Can you work these out from the model? Positions are in its coordinate system, mm. A direction names the side the tool comes from. Give positions to 0.01 mm unless a question says otherwise; leave off trailing zeros. Write each loop counter-clockwise with the first axis right and the second up, starting at its lowest first coordinate (ties: lowest second). Pieces come first, ordered by that corner, then holes. Notation, with made-up numbers: (5, -28) -> (48, -28) arc R15 ccw to (48, -20) -> close; hole circle Ø10 at (45.5, 88). An arc over 180 degrees is marked (long way). One line per item, written item: value.
from build123d import *

# Parameters (mm, degrees)
BOSS_EXTRUDE1_DEPTH     = 2.54
CUT_EXTRUDE1_DEPTH      = 60.34583774
CUT_EXTRUDE1_DEPTH_BACK = 60.34583774
SKETCH3_R               = 1.0922
SKETCH3_R_2             = 1.27
SKETCH3_R_3             = 1.016
SKETCH3_W               = 7.493
SKETCH3_H               = 35.56
SKETCH3_W_2             = 21.082
SKETCH3_H_2             = 21.59


with BuildPart() as part:
    # Sketch2 → Boss-Extrude1 (new body)
    with BuildSketch(Plane(origin=(0, 0, 0), x_dir=(1, 0, 0), z_dir=(0, 1, 0))):
        with BuildLine():
            Line((48.006, 34.798), (-48.006, 34.798))
            Line((-48.006, 34.798), (-48.006, -3.048))
            add(Edge.make_bspline(
                [(-48.006, -3.048), (-48.006, -45.381333333), (48.006, -45.381333333), (48.006, -3.048)],
                knots=[0, 0, 0, 0, 1, 1, 1, 1], degree=3))
            Line((48.006, -3.048), (48.006, 34.798))
        make_face()
    extrude(amount=BOSS_EXTRUDE1_DEPTH)

    # Sketch3 → Cut-Extrude1 (cut, two sides: drawn at the far end of the back side and taken through both)
    with BuildSketch(Plane(origin=(0, 2.54, 0), x_dir=(1, 0, 0), z_dir=(0, 1, 0)).offset(-CUT_EXTRUDE1_DEPTH_BACK)):
        with Locations(Location((-30.861, 23.4696, 0), (0, 0, 270))):
            Circle(SKETCH3_R)
        with Locations(Location((-30.861, 5.4864, 0), (0, 0, 270))):
            Circle(SKETCH3_R)
        with Locations(Location((-30.226, 30.988, 0), (0, 0, 270))):
            Circle(SKETCH3_R_2)
        with Locations(Location((30.861, 5.4864, 0), (0, 0, 90))):
            Circle(SKETCH3_R)
        with Locations(Location((30.861, 23.4696, 0), (0, 0, 90))):
            Circle(SKETCH3_R)
        with Locations(Location((-30.226, -22.352, 0), (0, 0, 270))):
            Circle(SKETCH3_R_2)
        with Locations(Location((30.226, -22.352, 0), (0, 0, 90))):
            Circle(SKETCH3_R_2)
        with Locations(Location((30.226, 30.988, 0), (0, 0, 90))):
            Circle(SKETCH3_R_2)
        with Locations(Location((-7.747, -22.606, 0), (0, 0, 270))):
            Circle(SKETCH3_R_3)
        with Locations(Location((7.747, -22.606, 0), (0, 0, 90))):
            Circle(SKETCH3_R_3)
        with Locations(Location((-20.828, 30.226, 0), (0, 0, 270))):
            Circle(SKETCH3_R_2)
        with Locations(Location((-20.828, -28.194, 0), (0, 0, 270))):
            Circle(SKETCH3_R_2)
        with Locations(Location((20.828, -28.194, 0), (0, 0, 90))):
            Circle(SKETCH3_R_2)
        with Locations(Location((20.828, 30.226, 0), (0, 0, 90))):
            Circle(SKETCH3_R_2)
        with Locations((-41.7195, 14.478)):
            Rectangle(SKETCH3_W, SKETCH3_H)
        with Locations((41.7195, 14.478)):
            Rectangle(SKETCH3_W, SKETCH3_H)
        with Locations((0, 14.859)):
            Rectangle(SKETCH3_W_2, SKETCH3_H_2)
    extrude(amount=CUT_EXTRUDE1_DEPTH + CUT_EXTRUDE1_DEPTH_BACK, mode=Mode.SUBTRACT)


solid = part.part
1) We'd pull the mould along Z, two halves only. Please class faces 3 (the face through (-6.74, 1.25, 22.47)), 4 (the face through (-31.927, 1.252, -5.723)), 5 (the face through (-1, 0, 5)): released by +Z, released by -Z, zero draft, split by the parting line, or undercut.
Answer list:
face 3: undercut
face 4: undercut
face 5: zero draft
2) If we section it at B-B (z = -16): Write out the boundary of the cut face in (x, y), and give its area (3 significant figures).
Answer list:
outline: (-48.01, 0) -> (-45.47, 0) -> (-45.47, 2.54) -> (-48.01, 2.54) -> close; (-37.97, 0) -> (-10.54, 0) -> (-10.54, 2.54) -> (-37.97, 2.54) -> close; (10.54, 0) -> (37.97, 0) -> (37.97, 2.54) -> (10.54, 2.54) -> close; (45.47, 0) -> (48.01, 0) -> (48.01, 2.54) -> (45.47, 2.54) -> close
area: 152 mm^2
3) If we section it at C-C (y = 0.9): State how many separate pieces and enclosed holes the cut face has, and give its area (3 significant figures).
Answer list:
separate pieces: 1
enclosed holes: 17
area: 5,020 mm^2
4) I need wall thicknesses on L1, parallel to X at y = 1.85, z = -22; L2, parallel to X at y = 2.1, z = -23.5; L3, parallel to X at y = 1, z = -28. Which ranges of each line are inside material? Lowest first, please.
Answer list:
L1: x = -48.01 to -45.47, -37.97 to -10.54, 10.54 to 37.97, 45.47 to 48.01
L2: x = -48.01 to -45.47, -37.97 to -31.95, -29.77 to -10.54, 10.54 to 29.77, 31.95 to 37.97, 45.47 to 48.01
L3: x = -48.01 to -45.47, -37.97 to 37.97, 45.47 to 48.01
5) If we section it at A-A (z = -3): Write out the boundary of the cut face in (x, y), and give its area (3 significant figures).
Answer list:
outline: (-48.01, 0) -> (-45.47, 0) -> (-45.47, 2.54) -> (-48.01, 2.54) -> close; (-37.97, 0) -> (37.97, 0) -> (37.97, 2.54) -> (-37.97, 2.54) -> close; (45.47, 0) -> (48.01, 0) -> (48.01, 2.54) -> (45.47, 2.54) -> close
area: 206 mm^2
6) Will this pin go through, and if not, where does the flat tip stop? pin 1 (1.5 mm diameter, centred on x = 10, y = 0.5, fed in from +Z).
Answer list:
pin 1: stops at z = 34.27
7) For faces 1 (the face through (10.541, 1, -15)), 2 (the face through (48.006, 1, -16)), which set-ups out of +Z, -Z, +X, -X, +Y, -Y let a thin tool reach every point of the face, with its end or its side?
Answer list:
face 1: +Y, -Y
face 2: +Z, -Z, +X, +Y, -Y
